Work out the finished part from the listing and answer in its coordinate system (mm). Face numbers are marked on the shaded views. A direction names the side the tool comes from. Give positions to 0.01 mm unless a question says otherwise; leave off trailing zeros. Loops run counter-clockwise (first coordinate to the right, second up) from the corner with the lowest first, then second, coordinate; pieces in that order, holes last. Notation, with made-up numbers: M -14.5,82.5 L 20.5,82.5 A21 ccw 20.5,94.5 Z; hole C 88,17.25 d4. An arc over 180 degrees is marked long. Answer as a JSON object with one key per item and string values. Group by question number.
```python
from build123d import *

# Parameters (mm, degrees)
SKETCH_1_W      = 22
SKETCH_1_H      = 28
SKETCH_1_R      = 1.3
EXTRUDE_1_DEPTH = 2
SKETCH_2_W      = 20
SKETCH_2_H      = 2.5
EXTRUDE_2_DEPTH = 10


with BuildPart() as part:
    # 草图1 → 凸台-拉伸1 (new body)
    with BuildSketch(Plane.XY):
        Rectangle(SKETCH_1_W, SKETCH_1_H)
        with Locations((-9, -11.997945994)):
            Circle(SKETCH_1_R, mode=Mode.SUBTRACT)
        with Locations((-9, -0.997945994)):
            Circle(SKETCH_1_R, mode=Mode.SUBTRACT)
        with Locations((9, -0.997945994)):
            Circle(SKETCH_1_R, mode=Mode.SUBTRACT)
        with Locations((9, -11.997945994)):
            Circle(SKETCH_1_R, mode=Mode.SUBTRACT)
    extrude(amount=EXTRUDE_1_DEPTH)

    # 草图2 → 凸台-拉伸2 (add)
    with BuildSketch(Plane.XY.offset(2)):
        with Locations((0, 11.25)):
            Rectangle(SKETCH_2_W, SKETCH_2_H)
    extrude(amount=EXTRUDE_2_DEPTH)


solid = part.part
```
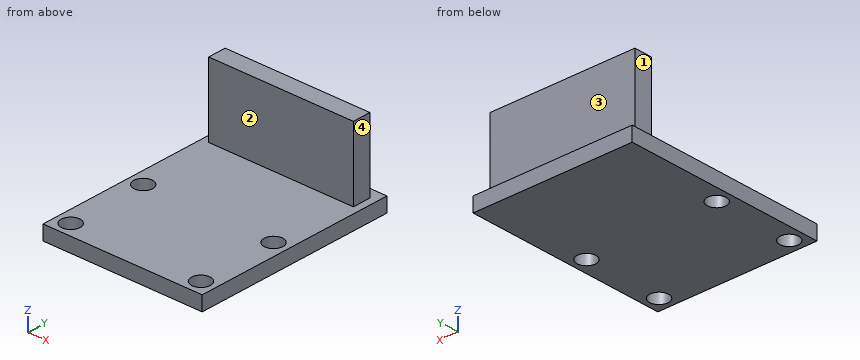
Item 1: Find the intervals of material crossed by probe 1 along Y at (x, z) = (-9, 1.65); probe 2 along Y at (x, z) = (1.25, 3.25); probe 3 along Z at (x, y) = (-2, -4), in increasing order. Write a range as [from, to].
Item 2: A cutting plane is placed at C-C (x = -4.75). Determine the outline of the cut face in (y, z), and give its area (3 significant figures).
Item 3: A tool of negligible diameter and unlimited length cuts with its end or side. For the marked faces 1, 2, 3 and 4, from which of +Z, -Z, +X, -X, +Y, -Y can it reach the whole face along a straight path? Write none if from no direction.
Item 4: A cutting plane is placed at A-A (x = 9). Determine the outline of the cut face in (y, z).
Item 5: Given pin 1 Ø2 at (y, z) = (10.5, 9.5) entering from -X; pin 2 Ø3 at (y, z) = (11.5, 9) entering from +X; pin 3 Ø2.5 at (x, y) = (9, -1) entering from -Z; pin 4 Ø4 at (x, z) = (6.5, 9) entering from +Y, each flat-ended and moving along its own axis, determine where each tip first touches the part or whether it passes through.
Item 6: A cutting plane is placed at D-D (z = 6.75). Determine the outline of the cut face in (x, y), and give its area (3 significant figures).
Item 7: A cutting plane is placed at B-B (y = -3). Determine the outline of the cut face in (x, z), and give its area (3 significant figures).
The answers:
{
 "1": {"probe 1": "y = [-14, -13.3], [-10.7, -2.3], [0.3, 14]", "probe 2": "y = [10, 12.5]", "probe 3": "z = [0, 2]"},
 "2": {"outline": "M -14,0 L 14,0 L 14,2 L 12.5,2 L 12.5,12 L 10,12 L 10,2 L -14,2 Z", "area": "81.0 mm^2"},
 "3": {"face 1": "+Z, -X, +Y, -Y", "face 2": "+Z, +X, -X, -Y", "face 3": "+Z, +X, -X, +Y", "face 4": "+Z, +X, +Y, -Y"},
 "4": {"outline": "M -14,0 L -13.3,0 L -13.3,2 L -14,2 Z; M -10.7,0 L -2.3,0 L -2.3,2 L -10.7,2 Z; M 0.3,0 L 14,0 L 14,2 L 12.5,2 L 12.5,12 L 10,12 L 10,2 L 0.3,2 Z"},
 "5": {"pin 1": "stops at x = -10", "pin 2": "stops at x = 10", "pin 3": "passes through", "pin 4": "stops at y = 12.5"},
 "6": {"outline": "M -10,10 L 10,10 L 10,12.5 L -10,12.5 Z", "area": "50.0 mm^2"},
 "7": {"outline": "M -11,0 L 11,0 L 11,2 L -11,2 Z", "area": "44.0 mm^2"}
}
